Can you work these out from the model? Positions are in its coordinate system, mm. Face numbers are marked on the shaded views. Give positions to 0.01 mm unless a question says otherwise; leave off trailing zeros. Order: outer loops, then holes, each group sorted by start corner. A loop starts at its lowest first (then second) coordinate and runs counter-clockwise, first axis right, second up. Notation, with made-up numbers: (7, 30) -> (42, 30) arc R19 cw to (42, 36) -> close; hole circle Ø10 at (89, 47). An arc over 180 degrees is marked (long way). Answer as CSV lines item,"result".
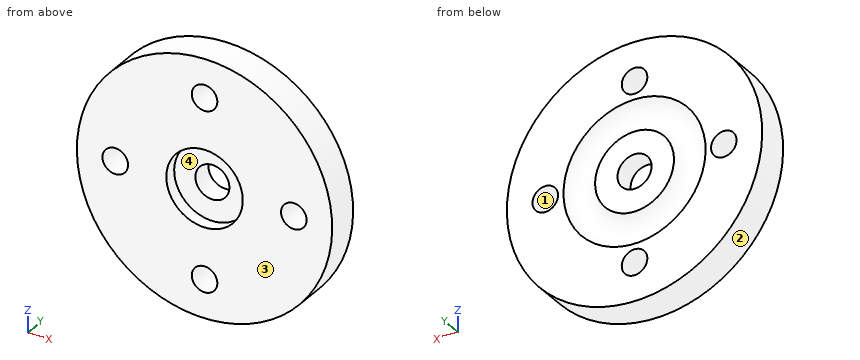
```python
from build123d import *

# Parameters (mm, degrees)
SKETCH1_R          = 11.9126
SKETCH1_R_2        = 1.1938
SKETCH1_R_3        = 6.7437
SKETCH1_R_4        = 5.1562
SKETCH1_R_5        = 3.5687
SKETCH1_R_6        = 1.5875
EXTRUDE1_DEPTH     = 3.175
SKETCH3_R          = 1.5875
CUT_EXTRUDE1_START = -1.9812
SKETCH1_3_R        = 3.5687
SKETCH1_3_R_2      = 1.5875
CUT_EXTRUDE1_DEPTH = 3.175
SKETCH1_4_R        = 1.5875
CUT_EXTRUDE2_DEPTH = 3.175


with BuildPart() as part:
    # Sketch1 → Extrude1 (new body)
    with BuildSketch(Plane(origin=(0, 0, 0), x_dir=(1, 0, 0), z_dir=(0, 1, 0))):
        with Locations(Location((0, 0, 0), (0, 0, 270))):  # turned: the seam where the file's is
            Circle(SKETCH1_R)
        with Locations(Location((-8.3312, 0, 0), (0, 0, 270))):  # turned: the seam where the file's is
            Circle(SKETCH1_R_2, mode=Mode.SUBTRACT)
        with Locations(Location((0, -8.3312, 0), (0, 0, 270))):  # turned: the seam where the file's is
            Circle(SKETCH1_R_2, mode=Mode.SUBTRACT)
        with Locations(Location((8.3312, 0, 0), (0, 0, 270))):  # turned: the seam where the file's is
            Circle(SKETCH1_R_2, mode=Mode.SUBTRACT)
        with Locations(Location((0, 8.3312, 0), (0, 0, 270))):  # turned: the seam where the file's is
            Circle(SKETCH1_R_2, mode=Mode.SUBTRACT)
        Circle(SKETCH1_R_3, mode=Mode.SUBTRACT)
        Circle(SKETCH1_R_3)
        Circle(SKETCH1_R_4, mode=Mode.SUBTRACT)
        Circle(SKETCH1_R_4)
        Circle(SKETCH1_R_5, mode=Mode.SUBTRACT)
        Circle(SKETCH1_R_5)
        Circle(SKETCH1_R_6, mode=Mode.SUBTRACT)
        Circle(SKETCH1_R_6)
    extrude(amount=-EXTRUDE1_DEPTH)

    # Sketch3 → Cut-Revolve1 (revolve, cut)
    with BuildSketch(Plane.XY, mode=Mode.PRIVATE) as cut_revolve1_sk:
        with Locations((5.1562, 0.5842)):
            Circle(SKETCH3_R)
    revolve(cut_revolve1_sk.sketch.rotate(Axis((0, 5.548517396, 0), (0, -1, 0)), 90), axis=Axis((0, 5.548517396, 0), (0, -1, 0)), mode=Mode.SUBTRACT)  # turned: the seam where the file's is

    # Sketch1_3 → Cut-Extrude1 (cut)
    with BuildSketch(Plane(origin=(0, 0, 0), x_dir=(1, 0, 0), z_dir=(0, 1, 0)).offset(CUT_EXTRUDE1_START)):
        with Locations(Location((0, 0, 0), (0, 0, 270))):  # turned: the seam where the file's is
            Circle(SKETCH1_3_R)
        Circle(SKETCH1_3_R_2, mode=Mode.SUBTRACT)
        Circle(SKETCH1_3_R_2)
    extrude(amount=-CUT_EXTRUDE1_DEPTH, mode=Mode.SUBTRACT)

    # Sketch1_4 → Cut-Extrude2 (cut)
    with BuildSketch(Plane(origin=(0, 0, 0), x_dir=(1, 0, 0), z_dir=(0, 1, 0))):
        with Locations(Location((0, 0, 0), (0, 0, 270))):  # turned: the seam where the file's is
            Circle(SKETCH1_4_R)
    extrude(amount=-CUT_EXTRUDE2_DEPTH, mode=Mode.SUBTRACT)


solid = part.part
```
Item 1: Imagine slicing it at C-C, the plane y = -0.3. Please give me the cut outline in (x, z) (1 decimal), then the cut area to 3 significant figures.
Numbers:
outline,"circle Ø23.8 at (0, 0); circle Ø7.7 at (0, 0); hole circle Ø2.4 at (-8.3, 0); hole circle Ø12.9 at (0, 0); hole circle Ø3.2 at (0, 0); hole circle Ø2.4 at (0, -8.3); hole circle Ø2.4 at (0, 8.3); hole circle Ø2.4 at (8.3, 0)"
area,"335 mm²"
Item 2: We'd pull the mould along X, two halves only. Please class the marked faces 1, 2, 3 and 4: released by +X, released by -X, zero draft, split by the parting line, or undercut.
Numbers:
face 1,"undercut"
face 2,"split by the parting line"
face 3,"zero draft"
face 4,"undercut"
Item 3: For pin 1 (2 mm diameter, centred on x = 8.33, z = 0, fed in from +Y); pin 2 (2 mm diameter, centred on x = -0.5, z = 1, fed in from -Y); pin 3 (1.5 mm diameter, centred on x = 2.5, y = -1, fed in from -Z), each with a flat end and sliding along its axis, tell me the tip position at first contact or that it passes through.
Numbers:
pin 1,"passes through"
pin 2,"stops at y = -1.98"
pin 3,"stops at z = -11.78"
Item 4: Imagine slicing it at B-B, the plane x = 0. Please give me the cut outline in (y, z) (1 decimal), then the cut area to 3 significant figures.
Numbers:
outline,"(-3.2, -11.9) -> (0, -11.9) -> (0, -9.5) -> (-3.2, -9.5) -> close; (-3.2, -7.1) -> (0, -7.1) -> (0, -6.6) arc R1.6 cw to (0, -3.7) -> (0, -1.6) -> (-2, -1.6) -> (-2, -3.6) -> (-3.2, -3.6) -> close; (-3.2, 3.6) -> (-2, 3.6) -> (-2, 1.6) -> (0, 1.6) -> (0, 3.7) arc R1.6 cw to (0, 6.6) -> (0, 7.1) -> (-3.2, 7.1) -> close; (-3.2, 9.5) -> (0, 9.5) -> (0, 11.9) -> (-3.2, 11.9) -> close"
area,"41.4 mm²"
Item 5: Please list where these lines run through material, in increasing order: line 1 along Z through (x, y) = (-1, -0.3); line 2 along X through (y, z) = (-2.3, 0) (3 decimals); line 3 along X through (y, z) = (-0.6, 0) (1 decimal).
Numbers:
line 1,"z = -11.87 to -8.98, -7.68 to -6.4, -3.71 to -1.23, 1.23 to 3.71, 6.4 to 7.68, 8.98 to 11.87"
line 2,"x = -11.913 to -9.525, -7.137 to -3.569, 3.569 to 7.137, 9.525 to 11.913"
line 3,"x = -11.9 to -9.5, -7.1 to -6.2, -4.1 to -1.6, 1.6 to 4.1, 6.2 to 7.1, 9.5 to 11.9"
Item 6: Imagine slicing it at A-A, the plane z = 0. Please give me the cut outline in (x, y) (1 decimal).
Numbers:
outline,"(-11.9, -3.2) -> (-9.5, -3.2) -> (-9.5, 0) -> (-11.9, 0) -> close; (-7.1, -3.2) -> (-3.6, -3.2) -> (-3.6, -2) -> (-1.6, -2) -> (-1.6, 0) -> (-3.7, 0) arc R1.6 cw to (-6.6, 0) -> (-7.1, 0) -> close; (1.6, -2) -> (3.6, -2) -> (3.6, -3.2) -> (7.1, -3.2) -> (7.1, 0) -> (6.6, 0) arc R1.6 cw to (3.7, 0) -> (1.6, 0) -> close; (9.5, -3.2) -> (11.9, -3.2) -> (11.9, 0) -> (9.5, 0) -> close"
Item 7: Imagine slicing it at D-D, the plane y = -2.4. Please give me the cut outline in (x, z) (3 decimals), then the cut area to 3 significant figures.
Numbers:
outline,"circle Ø23.825 at (0, 0); hole circle Ø2.388 at (-8.331, 0); hole circle Ø7.137 at (0, 0); hole circle Ø2.388 at (0, -8.331); hole circle Ø2.388 at (0, 8.331); hole circle Ø2.388 at (8.331, 0)"
area,"388 mm²"
